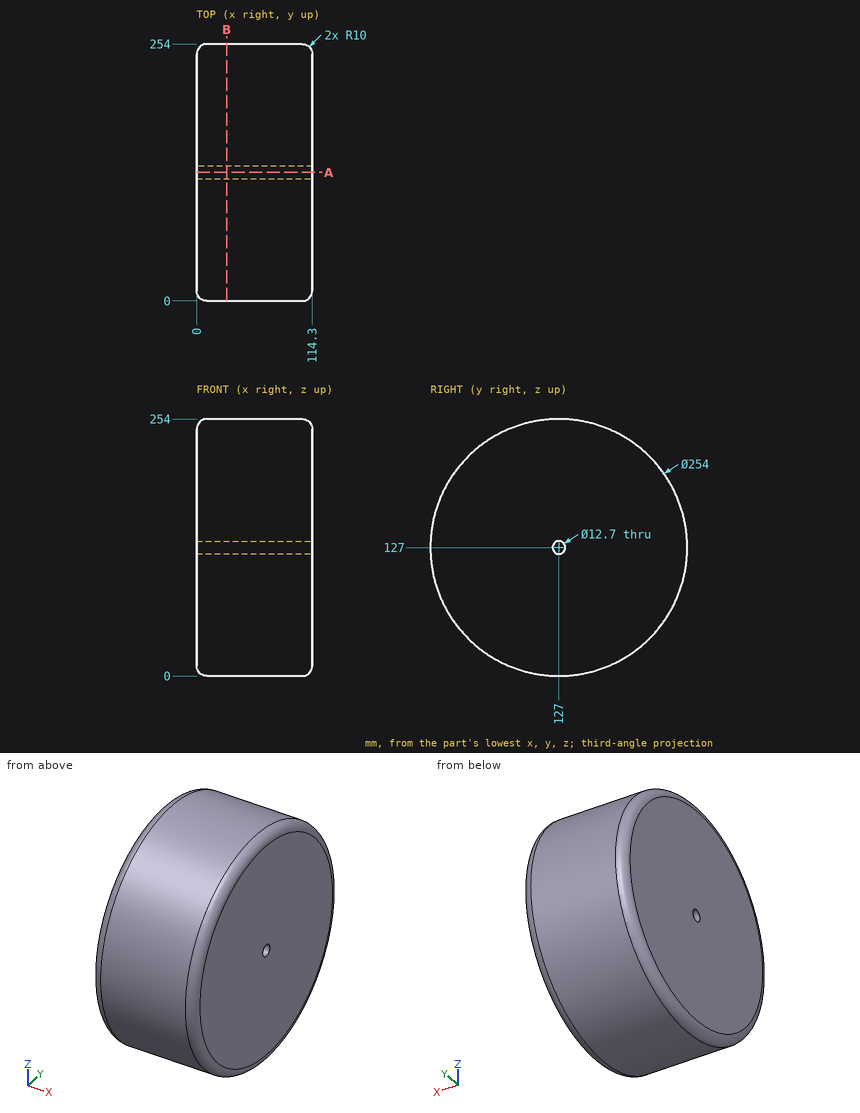
The figure shows three views and two pictorial views of one solid part (mm, origin at its lowest corner). Answer the questions. Round coordinates to 2 decimals unless told otherwise and drop trailing zeros. Loops run counter-clockwise (first coordinate to the right, second up) from the corner with the lowest first, then second, coordinate; pieces in that order, holes last. Notation, with made-up numbers: (-27, 5) -> (-8, 5) arc R27 ccw to (-8, 43) -> close; hole circle Ø6 at (30.5, 76). An arc over 180 degrees is marked (long way). Use one line per item in the form item = value.
(1) Find section B-B on x = 29.5. Give the vertices of the cut face in (y, z), then the cut area to 3 significant figures.
Answer list:
outline = circle Ø254 at (127, 127); hole circle Ø12.7 at (127, 127)
area = 50,500 mm2
(2) Flat-ended cylindrical pins translate along their axes: P1, Ø8, axis at x = 11.5, z = 221.5, coming from the -Y side; P2, Ø10, axis at x = 13, y = 185.5, coming from the +Z side; P3, Ø2, axis at x = 21.5, z = 62.5, coming from the -Y side. Find the tip coordinate at first contact, or state that the pin passes through.
Answer list:
P1 = 37.9
P2 = 242.18
P3 = 17.01
(3) Find section A-A on y = 127. Give the vertices of the cut face in (x, z), then the cut area to 3 significant figures.
Answer list:
outline = (0, 10) arc R10 ccw to (10, 0) -> (104.3, 0) arc R10 ccw to (114.3, 10) -> (114.3, 120.65) -> (0, 120.65) -> close; (0, 133.35) -> (114.3, 133.35) -> (114.3, 244) arc R10 ccw to (104.3, 254) -> (10, 254) arc R10 ccw to (0, 244) -> close
area = 27,500 mm2
(4) Straight lines are drawn through the part: line 1 (Z direction, x = 35, y = 127); line 2 (X direction, y = 243.5, z = 115.5); line 3 (Y direction, x = 57, z = 122). For each, find the intervals that lie inside material, in ascending order.
Answer list:
line_1 = 0 to 120.65, 133.35 to 254
line_2 = 0 to 114.3
line_3 = 0.1 to 123.09, 130.91 to 253.9
